Input: part model. Units: mm. Frame: model coordinates. A direction names the side the tool comes from. Round coordinates to 2 decimals unless told otherwise and drop trailing zeros. Write each loop counter-clockwise with the first axis right and the second up, starting at its lowest first coordinate (ties: lowest second). Pieces come first, ordered by that corner, then holes. Notation, with made-up numbers: (-10, 63.5) -> (31, 63.5) arc R17 cw to (31, 80.5) -> close; hole circle Ø8 at (51.25, -26). An arc over 180 degrees is marked (long way). Write item = value, one per line.
```python
from build123d import *

# Parameters (mm, degrees)
SKETCH1_R           = 2.45
BOSS_EXTRUDE2_DEPTH = 7.9
CUT_EXTRUDE1_DEPTH  = 7.9
CUT_EXTRUDE2_DEPTH  = 7.9


with BuildPart() as part:
    # Sketch1 → Boss-Extrude2 (new body)
    with BuildSketch(Plane(origin=(0, 0, 0), x_dir=(1, 0, 0), z_dir=(0, 1, 0))):
        with BuildLine():
            Line((52.027202313, -12.303856257), (37.545386148, 2.177959908))
            ThreePointArc((37.545386148, 2.177959908), (36.40113067, 3.042915189), (35, 3.35))
            Line((35, 3.35), (0, 3.35))
            ThreePointArc((0, 3.35), (-3.35, 0), (0, -3.35))
            Line((0, -3.35), (33.72619107, -3.098372284))
            Line((33.72619107, -3.098372284), (47.353836826, -17.084292963))
            ThreePointArc((47.353836826, -17.084292963), (52.244724969, -17.191071452), (52.027202313, -12.303856257))
        make_face()
        with Locations(Location((44.899494937, -9.899494937, 0), (0, 0, 270))):
            Circle(SKETCH1_R, mode=Mode.SUBTRACT)
        with Locations(Location((39.949747468, -4.949747468, 0), (0, 0, 270))):
            Circle(SKETCH1_R, mode=Mode.SUBTRACT)
        with Locations(Location((7, 0, 0), (0, 0, 270))):
            Circle(SKETCH1_R, mode=Mode.SUBTRACT)
        with Locations(Location((14, 0, 0), (0, 0, 270))):
            Circle(SKETCH1_R, mode=Mode.SUBTRACT)
        with Locations(Location((21, 0, 0), (0, 0, 270))):
            Circle(SKETCH1_R, mode=Mode.SUBTRACT)
        with Locations(Location((35, 0, 0), (0, 0, 270))):
            Circle(SKETCH1_R, mode=Mode.SUBTRACT)
        with Locations(Location((28, 0, 0), (0, 0, 270))):
            Circle(SKETCH1_R, mode=Mode.SUBTRACT)
    extrude(amount=BOSS_EXTRUDE2_DEPTH)

    # Sketch2 → Cut-Extrude1 (cut)
    with BuildSketch(Plane(origin=(0, 7.9, 0), x_dir=(1, 0, 0), z_dir=(0, 1, 0))):
        Polygon((0, 2.4), (0, 0), (0, -2.4), (0.9, -2.4), (0.9, -0.9), (2.4, -0.9), (2.4, 0.9), (0.9, 0.9), (0.9, 2.4), align=None)
        Polygon((-2.4, 0), (0, 0), (0, 2.4), (-0.9, 2.4), (-0.9, 0.9), (-2.4, 0.9), align=None)
        Polygon((0, -2.4), (0, 0), (-2.4, 0), (-2.4, -0.9), (-0.9, -0.9), (-0.9, -2.4), align=None)
    extrude(amount=-CUT_EXTRUDE1_DEPTH, mode=Mode.SUBTRACT)

    # Sketch3 → Cut-Extrude2 (cut)
    with BuildSketch(Plane(origin=(0, 7.9, 0), x_dir=(1, 0, 0), z_dir=(0, 1, 0))):
        Polygon((49.704933947, -15.966785192), (49.061371467, -15.33763709), (48.010311985, -16.412777338), (48.653874465, -17.041925441), align=None)
        Polygon((48.010311985, -16.412777338), (49.061371467, -15.33763709), (48.417808987, -14.708488988), (47.366749505, -15.783629236), align=None)
        Polygon((49.061371467, -15.33763709), (49.690519569, -14.69407461), (49.04695709, -14.064926508), (48.417808987, -14.708488988), align=None)
        Polygon((50.334082049, -15.323222713), (49.690519569, -14.69407461), (49.061371467, -15.33763709), (49.704933947, -15.966785192), align=None)
        Polygon((51.368247842, -16.334225476), (50.334082049, -15.323222713), (49.704933947, -15.966785192), (50.73909974, -16.977787956), align=None)
        Polygon((51.997395944, -15.690662997), (50.963230152, -14.679660233), (50.334082049, -15.323222713), (51.368247842, -16.334225476), align=None)
        Polygon((50.963230152, -14.679660233), (50.319667672, -14.05051213), (49.690519569, -14.69407461), (50.334082049, -15.323222713), align=None)
        Polygon((52.014289634, -13.604519984), (51.370727154, -12.975371882), (50.319667672, -14.05051213), (50.963230152, -14.679660233), align=None)
        Polygon((50.319667672, -14.05051213), (51.370727154, -12.975371882), (50.727164674, -12.34622378), (49.676105192, -13.421364028), align=None)
        Polygon((49.690519569, -14.69407461), (50.319667672, -14.05051213), (49.676105192, -13.421364028), (49.04695709, -14.064926508), align=None)
        Polygon((49.04695709, -14.064926508), (49.676105192, -13.421364028), (48.641939399, -12.410361264), (48.012791297, -13.053923744), align=None)
        Polygon((48.417808987, -14.708488988), (49.04695709, -14.064926508), (48.012791297, -13.053923744), (47.383643195, -13.697486224), align=None)
    extrude(amount=-CUT_EXTRUDE2_DEPTH, mode=Mode.SUBTRACT)


solid = part.part
```
1) Cut plane B-B (x = 28). Return the cut outline in (y, z), and give its area (3 significant figures).
Solutions:
outline = (0, -3.35) -> (7.9, -3.35) -> (7.9, -2.45) -> (0, -2.45) -> close; (0, 2.45) -> (7.9, 2.45) -> (7.9, 3.14) -> (0, 3.14) -> close
area = 12.6 mm^2
2) Cut plane C-C (z = 5.25). Return the cut outline in (x, y).
Solutions:
outline = (35.82, 0) -> (37.52, 0) -> (37.52, 7.9) -> (35.82, 7.9) -> close; (42.38, 0) -> (44.97, 0) -> (44.97, 7.9) -> (42.38, 7.9) -> close
3) Cut plane D-D (y = 1.75). Count the separate pieces of the cut face and the enclosed holes in it, and give its area (3 significant figures).
Solutions:
separate_pieces = 1
enclosed_holes = 9
area = 243 mm^2
4) Draft query along Z for faces 1 (the face through (25, 0, 3)), 2 (the face through (40.44, 3.89, 9.99)), 3 (the face through (48.022, 4.005, 13.045)). Return one class per face: +Z half, -Z half, draft (parallel to the pull), parting line (faces both ways), or undercut.
Solutions:
face_1 = draft
face_2 = +Z half
face_3 = undercut
5) First-contact query: P1, Ø2, axis at x = 35, y = 2, coming from the +Z side; P2, Ø0.8, axis at y = 5.5, z = 2, coming from the +X side; P3, Ø0.9, axis at x = 0, y = 3.5, coming from the +Z side; P4, Ø4, axis at x = 39.95, z = 4.95, coming from the -Y side. Flat tips, straight axial feed; report the tip coordinate or a pass-through.
Solutions:
P1 = 5.43
P2 = 42.12
P3 = 3.35
P4 = through
6) Cut plane A-A (z = 0). Return the cut outline in (x, y).
Solutions:
outline = (-3.35, 0) -> (-2.4, 0) -> (-2.4, 7.9) -> (-3.35, 7.9) -> close; (2.4, 0) -> (4.55, 0) -> (4.55, 7.9) -> (2.4, 7.9) -> close; (9.45, 0) -> (11.55, 0) -> (11.55, 7.9) -> (9.45, 7.9) -> close; (16.45, 0) -> (18.55, 0) -> (18.55, 7.9) -> (16.45, 7.9) -> close; (23.45, 0) -> (25.55, 0) -> (25.55, 7.9) -> (23.45, 7.9) -> close; (30.45, 0) -> (32.55, 0) -> (32.55, 7.9) -> (30.45, 7.9) -> close; (37.45, 0) -> (39.72, 0) -> (39.72, 7.9) -> (37.45, 7.9) -> close
7) Access query for faces 4 (the face through (-0.9, 4, -2)), 5 (the face through (25, 7.9, 3)). Directions: +Z, -Z, +X, -X, +Y, -Y. A direction counts if a zero-diameter tool reaches every point of the face in a straight line with its end or side. Return the directions, or none.
Solutions:
face_4 = +Y, -Y
face_5 = +Z, -Z, +X, -X, +Y
8) Line query: L1, parallel to X at y = 2.25, z = 16.5; L2, parallel to Z at x = 48, y = 6.75; L3, parallel to X at y = 6.75, z = 16.25. Output: solid intervals per line, ascending. Write a range as from..to.
Solutions:
L1 = 46.78..48.1, 49.18..50.25, 51.21..52.76
L2 = 8.28..13.07, 14.3..15.14, 16.4..17.64
L3 = 46.54..47.84, 49.43..49.99, 51.45..52.89
